from build123d import *

# Parameters (mm, degrees)
EXTRUDE_1_DEPTH      = 120
EXTRUDE_1_DEPTH_BACK = 120
EXTRUDE_START        = 84
SKETCH_1_5_R         = 1.6
EXTRUDE_2_DEPTH      = 16
EXTRUDE_3_DEPTH      = 20
EXTRUDE_3_DEPTH_BACK = 20
CUT_EXTRUDE_1_REACH  = 148.454
SKETCH_3_W           = 40
SKETCH_3_H           = 34.471908326
SKETCH_3_H_2         = 5.528091674
SKETCH_4_R           = 1.5
CUT_EXTRUDE_2_DEPTH  = 147.454080652
EXTRUDE_START_2      = 35
SKETCH_5_W           = 2.5
SKETCH_5_H           = 2.5
EXTRUDE_4_DEPTH      = 40
CUT_EXTRUDE_3_REACH  = 148.454
SKETCH_6_W           = 40
SKETCH_6_H           = 19.615168576
SKETCH_7_W           = 30
SKETCH_7_H           = 16.35748171
CUT_EXTRUDE_4_DEPTH  = 2.5
SKETCH_8_R           = 1.6
CUT_EXTRUDE_5_DEPTH  = 2.5
SKETCH_9_R           = 1.6
CUT_EXTRUDE_6_DEPTH  = 4


with BuildPart() as part:
    # 草图1 → 凸台-拉伸1 (new, two sides: drawn at the far end of the back side and taken through both)
    with BuildSketch(Plane(origin=(0, 0, 0), x_dir=(0, 0, -1), z_dir=(1, 0, 0)).offset(-EXTRUDE_1_DEPTH_BACK)):
        with BuildLine():
            Line((-3.458804046, -0.535419994), (-62.760974675, -57.105691992))
            Line((-62.760974675, -57.105691992), (-60, -60))
            Line((-60, -60), (-0.697829371, -3.429728002))
            ThreePointArc((-0.697829371, -3.429728002), (-2.532519507, -2.41585284), (-3.458804046, -0.535419994))
        make_face()
        Polygon((-62.760974675, -57.105691992), (-65.795054966, -60), (-60, -60), align=None)
        with BuildLine():
            Line((-0.697829371, -3.429728002), (-3.458804046, -0.535419994))
            ThreePointArc((-3.458804046, -0.535419994), (-2.532519507, -2.41585284), (-0.697829371, -3.429728002))
        make_face()
    extrude(amount=EXTRUDE_1_DEPTH + EXTRUDE_1_DEPTH_BACK)

    # 草图1<5> → 凸台-拉伸2 (add)
    with BuildSketch(Plane(origin=(0, 0, 0), x_dir=(0, 0, -1), z_dir=(1, 0, 0)).offset(EXTRUDE_START)):
        with BuildLine():
            ThreePointArc((3.5, 0), (-0.268501246, 3.489685814), (-3.458804046, -0.535419994))
            Line((-3.458804046, -0.535419994), (-0.697829371, -3.429728002))
            ThreePointArc((-0.697829371, -3.429728002), (2.214452212, -2.710387684), (3.5, 0))
        make_face()
        Circle(SKETCH_1_5_R, mode=Mode.SUBTRACT)
    extrude_2 = extrude(amount=EXTRUDE_2_DEPTH)

    # 镜向1: 凸台-拉伸2 across plane
    add(extrude_2.mirror(Plane(origin=(0, 0, 0), x_dir=(0, 0, 1), z_dir=(1, 0, 0))))

    # 草图2 → 凸台-拉伸3 (add, two sides: drawn at the far end of the back side and taken through both)
    with BuildSketch(Plane(origin=(0, 0, 0), x_dir=(0, 0, -1), z_dir=(1, 0, 0)).offset(-EXTRUDE_3_DEPTH_BACK)):
        Polygon((-4.568589556, -7.12217221), (-7.068589556, -9.507003634), (-7.068589556, -43.97891196), (-43.205219579, -43.97891196), (-45.82594989, -46.47891196), (-4.568589556, -46.47891196), align=None)
    extrude(amount=EXTRUDE_3_DEPTH + EXTRUDE_3_DEPTH_BACK)

    # 切除-拉伸1: up to this face of the body (flat: up to its plane)
    cut_extrude_1_end = Plane(part.part.faces().sort_by_distance((0, -30.267709997, 34.626929506))[0])
    # 草图3 → 切除-拉伸1 (cut, up to the picked face)
    with BuildSketch(Plane.XY.offset(7.068589556), mode=Mode.PRIVATE) as cut_extrude_1_sk1:
        with Locations((0, -26.742957797)):
            Rectangle(SKETCH_3_W, SKETCH_3_H)
    cut_extrude_1_tool1 = split(extrude(cut_extrude_1_sk1.sketch, amount=CUT_EXTRUDE_1_REACH, mode=Mode.PRIVATE), bisect_by=cut_extrude_1_end, keep=Keep.BOTH, mode=Mode.PRIVATE)
    # 草图3 → 切除-拉伸1 (cut, up to the picked face)
    with BuildSketch(Plane.XY.offset(7.068589556), mode=Mode.PRIVATE) as cut_extrude_1_sk2:
        with Locations((0, -6.742957797)):
            Rectangle(SKETCH_3_W, SKETCH_3_H_2)
    cut_extrude_1_tool2 = split(extrude(cut_extrude_1_sk2.sketch, amount=CUT_EXTRUDE_1_REACH, mode=Mode.PRIVATE), bisect_by=cut_extrude_1_end, keep=Keep.BOTH, mode=Mode.PRIVATE)
    add(cut_extrude_1_tool1.solids().sort_by(Axis((0, -26.742958, 7.06859), (0, 0, 1)))[0], mode=Mode.SUBTRACT)
    add(cut_extrude_1_tool2.solids().sort_by(Axis((0, -6.742958, 7.06859), (0, 0, 1)))[0], mode=Mode.SUBTRACT)

    # 草图4 → 切除-拉伸2 (cut, through all)
    with BuildSketch(Plane.XY.offset(7.068589556)):
        with Locations((-17, -6.97891196)):
            Circle(SKETCH_4_R)
        with Locations((17, -6.97891196)):
            Circle(SKETCH_4_R)
        with Locations((17, -40.97891196)):
            Circle(SKETCH_4_R)
        with Locations((-17, -40.97891196)):
            Circle(SKETCH_4_R)
    extrude(amount=-CUT_EXTRUDE_2_DEPTH, mode=Mode.SUBTRACT)

    # 草图5 → 凸台-拉伸4 (add)
    with BuildSketch(Plane(origin=(0, 0, 0), x_dir=(0, 0, -1), z_dir=(1, 0, 0)).offset(EXTRUDE_START_2)):
        Polygon((-27.6310163, -29.12217221), (-30.251746612, -31.62217221), (-7.068589556, -31.62217221), (-7.068589556, -29.12217221), align=None)
        Polygon((-7.068589556, -29.12217221), (-4.568589556, -29.12217221), (-4.568589556, -7.12217221), (-7.068589556, -9.507003634), align=None)
        with Locations((-5.818589556, -30.37217221)):
            Rectangle(SKETCH_5_W, SKETCH_5_H)
    extrude_4 = extrude(amount=EXTRUDE_4_DEPTH)

    # 切除-拉伸3: up to this plane
    cut_extrude_3_end = Plane(origin=(-120, 1.447154004, 1.380487337), z_dir=(0, -0.7235770020149496, -0.6902436686816169))
    # 草图6 → 切除-拉伸3 (cut, up to the surface)
    with BuildSketch(Plane.XY.offset(7.068589556), mode=Mode.PRIVATE) as cut_extrude_3_sk1:
        with Locations((55, -19.314587922)):
            Rectangle(SKETCH_6_W, SKETCH_6_H)
    cut_extrude_3_tool1 = split(extrude(cut_extrude_3_sk1.sketch, amount=CUT_EXTRUDE_3_REACH, mode=Mode.PRIVATE), bisect_by=cut_extrude_3_end, keep=Keep.BOTH, mode=Mode.PRIVATE)
    cut_extrude_3 = cut_extrude_3_tool1.solids().sort_by_distance((55, -19.314588, 7.06859))[0]
    add(cut_extrude_3, mode=Mode.SUBTRACT)

    # 草图7 → 切除-拉伸4 (cut)
    with BuildSketch(Plane(origin=(0, -29.12217221, 0), x_dir=(1, 0, 0), z_dir=(0, 1, 0))):
        with Locations((55, -15.247330411)):
            Rectangle(SKETCH_7_W, SKETCH_7_H)
    cut_extrude_4 = extrude(amount=-CUT_EXTRUDE_4_DEPTH, mode=Mode.SUBTRACT)

    # 草图8 → 切除-拉伸5 (cut)
    with BuildSketch(Plane.XY.offset(7.068589556)):
        with Locations((40.5, -21.12217221)):
            Circle(SKETCH_8_R)
        with Locations((69.5, -21.12217221)):
            Circle(SKETCH_8_R)
    cut_extrude_5 = extrude(amount=-CUT_EXTRUDE_5_DEPTH, mode=Mode.SUBTRACT)

    # 镜向2: 凸台-拉伸4 across plane
    add(extrude_4.mirror(Plane(origin=(0, 0, 0), x_dir=(0, 0, 1), z_dir=(1, 0, 0))))

    # 镜向3: 切除-拉伸4 across plane
    add(cut_extrude_4.mirror(Plane(origin=(0, 0, 0), x_dir=(0, 0, 1), z_dir=(1, 0, 0))), mode=Mode.SUBTRACT)

    # 镜向4: 切除-拉伸5 across plane
    add(cut_extrude_5.mirror(Plane(origin=(0, 0, 0), x_dir=(0, 0, 1), z_dir=(1, 0, 0))), mode=Mode.SUBTRACT)

    # 镜向5: 切除-拉伸3 across plane
    add(cut_extrude_3.mirror(Plane(origin=(0, 0, 0), x_dir=(0, 0, 1), z_dir=(1, 0, 0))), mode=Mode.SUBTRACT)

    # 草图9 → 切除-拉伸6 (cut)
    with BuildSketch(Plane(origin=(0, -1.447154004, -1.380487337), x_dir=(1, 0, 0), z_dir=(0, -0.7235770020149502, -0.6902436686816162))):
        with Locations(Location((113.511233503, 46.629240242, 0), (0, 0, 270))):
            Circle(SKETCH_9_R)
        with Locations(Location((92.317392528, 46.629240242, 0), (0, 0, 270))):
            Circle(SKETCH_9_R)
        with Locations(Location((-90.488766497, 46.629240242, 0), (0, 0, 270))):
            Circle(SKETCH_9_R)
        with Locations(Location((-111.682607472, 46.629240242, 0), (0, 0, 270))):
            Circle(SKETCH_9_R)
    extrude(amount=-CUT_EXTRUDE_6_DEPTH, mode=Mode.SUBTRACT)


solid = part.part
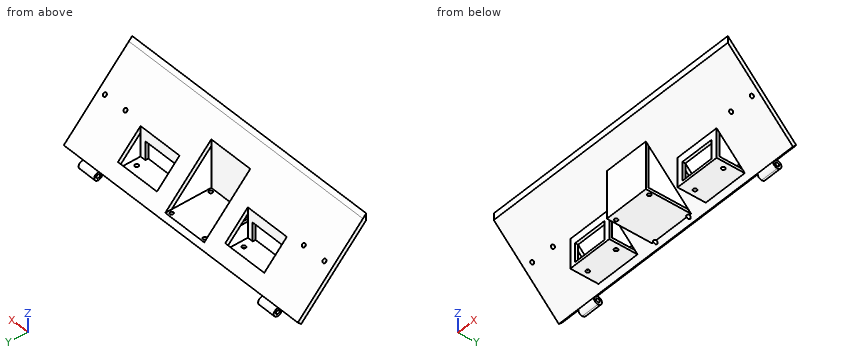
Here's how the part is built. I have some questions about the finished solid (model axes, mm). Round coordinates to 2 decimals unless told otherwise and drop trailing zeros. Write each loop counter-clockwise with the first axis right and the second up, starting at its lowest first coordinate (ties: lowest second). Pieces come first, ordered by that corner, then holes. Notation, with made-up numbers: (26.5, 69.25) -> (35.5, 69.25) arc R17 ccw to (35.5, 99.25) -> close; hole circle Ø11 at (-37, -16.75). An arc over 180 degrees is marked (long way). One line per item, written item: value.
1) Suppose I cut it at A-A on x = -46. List the corners of the cut face in (y, z) for me.
Filled sheet:
outline: (-60, 60) -> (-31.62, 30.25) -> (-31.62, 23.43) -> (-29.12, 23.43) -> (-29.12, 33.43) -> (-60, 65.8) -> close; (-31.62, 4.57) -> (-7.12, 4.57) -> (-3.43, 0.7) -> (-0.54, 3.46) -> (-9.51, 12.86) -> (-9.51, 7.07) -> (-31.62, 7.07) -> close
2) Suppose I cut it at C-C on z = 10. Give the number of separate pieces and of enclosed holes in the cut face, plus the area to 3 significant figures.
Filled sheet:
separate pieces: 7
enclosed holes: 0
area: 1,030 mm2
3) Suppose I cut it at B-B on x = 0. List the corners of the cut face in (y, z) for me, plus the area to 3 significant figures.
Filled sheet:
outline: (-60, 60) -> (-46.48, 45.83) -> (-46.48, 4.57) -> (-7.12, 4.57) -> (-3.43, 0.7) -> (-0.54, 3.46) -> (-3.98, 7.07) -> (-43.98, 7.07) -> (-43.98, 49) -> (-60, 65.8) -> close
area: 309 mm2
4) I'm going to push flat-ended pins straight in: pin 1 Ø7.5 at (y, z) = (-19.5, 11) entering from +X; pin 2 Ø3.5 at (y, z) = (1, -1) entering from +X; pin 3 Ø5 at (x, z) = (-42, 49) entering from +Y; pin 4 Ø6 at (x, z) = (59.5, 10.5) entering from -Y. Where does each tip first touch, or does it pass through?
Filled sheet:
pin 1: passes through
pin 2: stops at x = 100
pin 3: stops at y = -41.59
pin 4: stops at y = -9.51
5) If I drill on line 1 (X direction, y = -15.5, z = 19); line 2 (X direction, y = -31, z = 14.5); line 3 (Y direction, x = 90, z = 0), over which ranges is the centre line in solid material (lowest first)? Write a range as [from, to].
Filled sheet:
line 1: x = [-120, -75], [-35, -20], [20, 35], [75, 120]
line 2: x = [-75, -70], [-40, -35], [35, 40], [70, 75]
line 3: y = [-3.5, -1.6], [1.6, 3.5]
